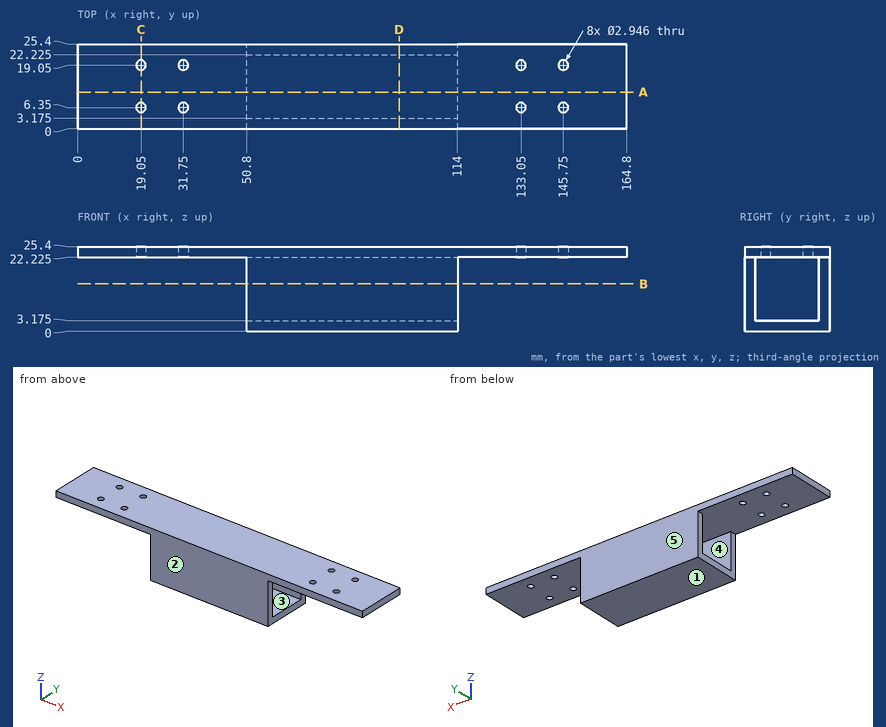
The drawing under review shows one solid part. Ordinate dimensions are in mm from its lowest x, y, z. A direction names the side the tool comes from. Round coordinates to 2 decimals unless told otherwise and drop trailing zeros. Loops run counter-clockwise (first coordinate to the right, second up) from the corner with the lowest first, then second, coordinate; pieces in that order, holes last. Notation, with made-up numbers: (-5, 40.25) - (17, 40.25) arc R25 ccw to (17, 78.25) - close; hole circle Ø11 at (22.5, 74.5). An arc over 180 degrees is marked (long way). One line per item, written item: value. Start each with the question number.
1) Draft analysis for pull direction Z (two halves, no side actions). For the marked faces 1, 2 and 3, state which applies: +Z half, -Z half, draft (parallel to the pull), parting line (faces both ways), or undercut.
2) Consider section C-C on x = 19.05. Give the boundary of the cut face in (y, z) (1 decimal).
3) For the marked faces 4 and 5, list the 3-axis set-ups (+Z, -Z, +X, -X, +Y, -Y) from which the entire face can be reached by the end or side of a thin tool; tool diameter is ignored.
4) Consider section D-D on x = 96.5. Give the boundary of the cut face in (y, z) (1 decimal).
5) Consider section B-B on z = 14.25. Give the boundary of the cut face in (x, y) (1 decimal).
6) Consider section A-A on y = 11. Give the boundary of the cut face in (x, z) (1 decimal), then the cut area to 3 significant figures.
7) Insertion check: pin 1 Ø6 at (y, z) = (14.5, 4.5) entering from +X; pin 2 Ø4 at (x, y) = (19.05, 19.05) entering from -Z (3 decimals); pin 3 Ø1.8 at (x, y) = (31.75, 6.35) entering from +Z. Each pin has a flat end and moves straight along its axis. Give the tip position at first contact, or say it passes through.
8) To check wall thickness, follow L1, parallel to Y at x = 133.05, z = 24.6; L2, parallel to Y at x = 65, z = 20.5 (1 decimal). State the ranges of each line that lie inside material, in increasing order. Write a range as from..to.
Reported:
1. face 1: -Z half
1. face 2: draft
1. face 3: undercut
2. outline: (0, 22.2) - (4.9, 22.2) - (4.9, 25.4) - (0, 25.4) - close; (7.8, 22.2) - (17.6, 22.2) - (17.6, 25.4) - (7.8, 25.4) - close; (20.5, 22.2) - (25.4, 22.2) - (25.4, 25.4) - (20.5, 25.4) - close
3. face 4: +X, -X
3. face 5: +Z, -Z, +X, -X, +Y
4. outline: (0, 0) - (25.4, 0) - (25.4, 25.4) - (0, 25.4) - close; hole (3.2, 3.2) - (22.2, 3.2) - (22.2, 22.2) - (3.2, 22.2) - close
5. outline: (50.8, 0) - (114, 0) - (114, 3.2) - (50.8, 3.2) - close; (50.8, 22.2) - (114, 22.2) - (114, 25.4) - (50.8, 25.4) - close
6. outline: (0, 22.2) - (164.8, 22.2) - (164.8, 25.4) - (0, 25.4) - close; (50.8, 0) - (114, 0) - (114, 3.2) - (50.8, 3.2) - close
6. area: 724 mm^2
7. pin 1: stops at x = 114
7. pin 2: stops at z = 22.225
7. pin 3: passes through
8. L1: y = 0..4.88, 7.82..17.58, 20.52..25.4
8. L2: y = 0..3.2, 22.2..25.4
